```python
from build123d import *
from OCP.BRepFilletAPI import BRepFilletAPI_MakeChamfer

# Parameters (mm, degrees)
SKETCH1_W           = 54
SKETCH1_H           = 10
BOSS_EXTRUDE1_DEPTH = 10.5
SKETCH2_R           = 2.15
CUT_EXTRUDE1_DEPTH  = 10.5
SKETCH3_W           = 4.3
SKETCH3_H           = 5
CUT_EXTRUDE2_DEPTH  = 10.5
CHAMFER3_SIZE       = 0.4
CHAMFER3_SIZE2      = 3
CHAMFER1_SIZE       = 2
CHAMFER2_SIZE       = 0.4
CHAMFER4_SIZE       = 0.4


with BuildPart() as part:
    # Sketch1 → Boss-Extrude1 (new body)
    with BuildSketch(Plane.XY):
        with Locations((27, 5)):
            Rectangle(SKETCH1_W, SKETCH1_H)
    extrude(amount=BOSS_EXTRUDE1_DEPTH)

    # Sketch2 → Cut-Extrude1 (cut)
    with BuildSketch(Plane.XY.offset(10.5)):
        with Locations((4.5, 5)):
            Circle(SKETCH2_R)
        with Locations((49.5, 5)):
            Circle(SKETCH2_R)
    extrude(amount=-CUT_EXTRUDE1_DEPTH, mode=Mode.SUBTRACT)

    # Sketch3 → Cut-Extrude2 (cut)
    with BuildSketch(Plane.XY.offset(10.5)):
        with Locations((4.5, 2.5)):
            Rectangle(SKETCH3_W, SKETCH3_H)
        with Locations((49.5, 2.5)):
            Rectangle(SKETCH3_W, SKETCH3_H)
    extrude(amount=-CUT_EXTRUDE2_DEPTH, mode=Mode.SUBTRACT)

    # Chamfer3: one chamfer whose edges measure the first distance from different faces: ONE call of the kernel's chamfer builder (chamfer() names one face for all edges)
    chamfer3_edges_1 = [part.edges().sort_by_distance(p)[0] for p in [
        (27, 0, 10.5),
    ]]
    chamfer3_side_1 = [part.faces().sort_by_distance(p)[0] for p in [
        (27, 0, 5.25),
    ]]
    chamfer3_edges_2 = [part.edges().sort_by_distance(p)[0] for p in [
        (52.825, 0, 10.5),
    ]]
    chamfer3_side_2 = [part.faces().sort_by_distance(p)[0] for p in [
        (52.825, 0, 5.25),
    ]]
    chamfer3_edges_3 = [part.edges().sort_by_distance(p)[0] for p in [
        (1.175, 0, 10.5),
    ]]
    chamfer3_side_3 = [part.faces().sort_by_distance(p)[0] for p in [
        (1.175, 0, 5.25),
    ]]
    chamfer3 = BRepFilletAPI_MakeChamfer(part.part.solid().wrapped)
    for e in chamfer3_edges_1:
        chamfer3.Add(CHAMFER3_SIZE, CHAMFER3_SIZE2, e.wrapped, chamfer3_side_1[0].wrapped)  # the first distance lies on this face
    for e in chamfer3_edges_2:
        chamfer3.Add(CHAMFER3_SIZE, CHAMFER3_SIZE2, e.wrapped, chamfer3_side_2[0].wrapped)  # the first distance lies on this face
    for e in chamfer3_edges_3:
        chamfer3.Add(CHAMFER3_SIZE, CHAMFER3_SIZE2, e.wrapped, chamfer3_side_3[0].wrapped)  # the first distance lies on this face
    add(Compound.cast(chamfer3.Shape()), mode=Mode.REPLACE)

    # Chamfer1
    chamfer1_edges = [part.edges().sort_by_distance(p)[0] for p in [
        (0, 0, 5.05),
        (54, 0, 5.05),
        (0, 10, 5.25),
        (54, 10, 5.25),
    ]]
    chamfer(chamfer1_edges, length=CHAMFER1_SIZE)

    # Chamfer2
    chamfer2_edges = [part.edges().sort_by_distance(p)[0] for p in [
        (49.5, 7.15, 10.5),
        (49.5, 7.15, 0),
        (4.5, 7.15, 10.5),
        (4.5, 7.15, 0),
        (51.65, 2.5, 0),
        (47.35, 2.5, 0),
        (51.65, 4, 10.5),
        (47.35, 4, 10.5),
        (6.65, 2.5, 0),
        (2.35, 2.5, 0),
        (6.65, 4, 10.5),
        (2.35, 4, 10.5),
    ]]
    chamfer(chamfer2_edges, length=CHAMFER2_SIZE)

    # Chamfer4
    # the kernel refuses this chamfer: 0.4 mm, written as the material it takes off along each edge
    with BuildSketch(Plane(origin=(47.35, 0, 11.128673195), x_dir=(-0.9996219169112968, -0.02749587661058673, 0), z_dir=(0, 0, -1)), Plane(origin=(2.35, 0, 11.128673195), x_dir=(-0.9996219169112968, -0.027495876610586386, 0), z_dir=(0, 0, -1))) as chamfer4_piece_1:
        Polygon((CHAMFER4_SIZE * 0.999621916911, CHAMFER4_SIZE * 0.0274958766106), (-CHAMFER4_SIZE * 0.0274958766106, CHAMFER4_SIZE * 0.999621916911), (0, 0), align=None)
    extrude(amount=11.75734639, mode=Mode.SUBTRACT)
    with BuildSketch(Plane(origin=(6.65, 0, 11.128673195), x_dir=(0.9996219169112968, -0.027495876610586324, 0), z_dir=(0, 0, -1)), Plane(origin=(51.65, 0, 11.128673195), x_dir=(0.9996219169112968, -0.02749587661058674, 0), z_dir=(0, 0, -1))) as chamfer4_piece_2:
        Polygon((CHAMFER4_SIZE * 0.999621916911, -CHAMFER4_SIZE * 0.0274958766106), (-CHAMFER4_SIZE * 0.0274958766106, -CHAMFER4_SIZE * 0.999621916911), (0, 0), align=None)
    extrude(amount=11.75734639, mode=Mode.SUBTRACT)


solid = part.part
```
CAD build for the part. Positions are in the model's coordinates, mm. A direction names the side the tool comes from. Give positions to 0.01 mm unless a question says otherwise; leave off trailing zeros. Order: outer loops, then holes, each group sorted by start corner. A loop starts at its lowest first (then second) coordinate and runs counter-clockwise, first axis right, second up. Notation, with made-up numbers: M -34.5,1 L 2.5,1 A16 ccw 2.5,20 Z; hole C 54,87.5 d7. An arc over 180 degrees is marked long. Put each result on its own line as item: value. Start each with the question number.
(1) Saw through at D-D, the plane y = 1.25. Write the cut outline in (x, z), then the cut area to 3 significant figures.
(2) Drill centre lines: line 1 along X through (y, z) = (3.25, 2.25); line 2 along X through (y, z) = (1.75, 1); line 3 along Y through (x, z) = (3, 1.5). Where is each one in solid material? Low to high.
(3) Which spindle directions (+Z, -Z, +X, -X, +Y, -Y) get a long thin tool onto all of the face, cutting with end or side? Do faces 1 (the flat face through (2.35, 3, 5)), 2 (the flat face through (1.14, 1.86, 10.35)). Say none if no direction does.
(4) Saw through at A-A, the plane y = 3.5. Write the cut outline in (x, z).
(5) Saw through at C-C, the plane x = 49.5. Write the cut outline in (y, z).
(6) Mould opens along Y. For faces 3 (the flat face through (1, 1, 5)), 4 (the flat face through (27, 10, 5)), 5 (the flat face through (0, 5, 5)) say: +Y half, -Y half, draft (parallel to the pull), parting line (faces both ways), or undercut.
(7) Saw through at B-B, the plane z = 1.25. Write the cut outline in (x, y) (3 decimals), then the cut area to 3 significant figures.
Check result:
1. outline: M 0.75,0 L 1.95,0 L 2.35,0.4 L 2.35,10.1 L 2.18,10.27 L 0.75,10.27 Z; M 6.65,0.4 L 7.05,0 L 46.95,0 L 47.35,0.4 L 47.35,10.1 L 47.18,10.27 L 6.82,10.27 L 6.65,10.1 Z; M 51.65,0.4 L 52.05,0 L 53.25,0 L 53.25,10.27 L 51.82,10.27 L 51.65,10.1 Z
1. area: 450 mm2
2. line 1: x = 0 to 2.35, 6.65 to 47.35, 51.65 to 54
2. line 2: x = 0.25 to 2.35, 6.65 to 47.35, 51.65 to 53.75
2. line 3: y = 6.54 to 10
3. face 1: +Z, -Z, -Y
3. face 2: +Z, +X, -X, -Y
4. outline: M 0,0 L 1.95,0 L 2.35,0.4 L 2.35,10.1 L 1.95,10.5 L 0,10.5 Z; M 6.65,0.4 L 7.05,0 L 46.95,0 L 47.35,0.4 L 47.35,10.1 L 46.95,10.5 L 7.05,10.5 L 6.65,10.1 Z; M 51.65,0.4 L 52.05,0 L 54,0 L 54,10.5 L 52.05,10.5 L 51.65,10.1 Z
5. outline: M 7.15,0.4 L 7.55,0 L 10,0 L 10,10.5 L 7.55,10.5 L 7.15,10.1 Z
6. face 3: -Y half
6. face 4: +Y half
6. face 5: draft
7. outline: M 0,2 L 1.975,0.025 L 2.35,0.4 L 2.35,5 A2.15 cw 6.65,5 L 6.65,0.4 L 7.05,0 L 46.95,0 L 47.35,0.4 L 47.35,5 A2.15 cw 51.65,5 L 51.65,0.4 L 52.025,0.025 L 54,2 L 54,8 L 52,10 L 2,10 L 0,8 Z
7. area: 474 mm2
